Can you work these out from the model? Positions are in its coordinate system, mm. Face numbers are marked on the shaded views. A direction names the side the tool comes from. Round coordinates to 2 decimals unless told otherwise and drop trailing zeros. Order: outer loops, then holes, each group sorted by start corner. A loop starts at its lowest first (then second) coordinate and runs counter-clockwise, first axis right, second up. Notation, with made-up numbers: M 70.5,54 L 81.5,54 A23 ccw 81.5,84 Z; hole C 20.5,-8 d1. An arc over 180 degrees is marked long. Answer as a JSON object with one key per item and string values. Group by question number.
from build123d import *

# Parameters (mm, degrees)
CROQUIS1_W              = 44
CROQUIS1_H              = 25
SALIENTE_EXTRUIR2_DEPTH = 10
CROQUIS2_W              = 42
CROQUIS2_H              = 23
CORTAR_EXTRUIR1_DEPTH   = 9
CROQUIS3_W              = 1
CROQUIS3_H              = 2
SALIENTE_EXTRUIR3_DEPTH = 25
CROQUIS4_W              = 42
CROQUIS4_H              = 23
CORTAR_EXTRUIR2_DEPTH   = 28
CROQUIS5_W              = 1
CROQUIS5_H              = 23
CORTAR_EXTRUIR10_DEPTH  = 5
CROQUIS6_W              = 29.89343235
CROQUIS6_H              = 11.447342814
CORTAR_EXTRUIR11_DEPTH  = 1
CROQUIS7_W              = 31.003837105
CROQUIS7_H              = 9.868746677
CORTAR_EXTRUIR12_DEPTH  = 1
CROQUIS8_W              = 1
CROQUIS8_H              = 23
SALIENTE_EXTRUIR4_DEPTH = 5
CROQUIS9_W              = 8
CROQUIS9_H              = 4
CORTAR_EXTRUIR17_DEPTH  = 87
CROQUIS10_R             = 4
CORTAR_EXTRUIR19_DEPTH  = 10


with BuildPart() as part:
    # Croquis1 → Saliente-Extruir2 (new body)
    with BuildSketch(Plane(origin=(0, 0, 0), x_dir=(1, 0, 0), z_dir=(0, 1, 0))):
        Rectangle(CROQUIS1_W, CROQUIS1_H)
    extrude(amount=SALIENTE_EXTRUIR2_DEPTH)

    # Croquis2 → Cortar-Extruir1 (cut)
    with BuildSketch(Plane(origin=(0, 10, 0), x_dir=(1, 0, 0), z_dir=(0, 1, 0))):
        Rectangle(CROQUIS2_W, CROQUIS2_H)
    extrude(amount=-CORTAR_EXTRUIR1_DEPTH, mode=Mode.SUBTRACT)

    # Croquis3 → Saliente-Extruir3 (add)
    with BuildSketch(Plane.XY.offset(12.5)):
        Polygon((-23, 10), (-22, 10), (-16, 10), (-20, 13.5), (-20, 15), (-23, 15), align=None)
        Polygon((20, 13.5), (16, 10), (22, 10), (23, 10), (23, 15), (20, 15), align=None)
        with Locations((-22.5, 9)):
            Rectangle(CROQUIS3_W, CROQUIS3_H)
        with Locations((22.5, 9)):
            Rectangle(CROQUIS3_W, CROQUIS3_H)
    extrude(amount=-SALIENTE_EXTRUIR3_DEPTH)

    # Croquis4 → Cortar-Extruir2 (cut)
    with BuildSketch(Plane(origin=(0, 1, 0), x_dir=(1, 0, 0), z_dir=(0, 1, 0))):
        Rectangle(CROQUIS4_W, CROQUIS4_H)
    extrude(amount=CORTAR_EXTRUIR2_DEPTH, mode=Mode.SUBTRACT)

    # Croquis5 → Cortar-Extruir10 (cut)
    with BuildSketch(Plane(origin=(0, 15, 0), x_dir=(1, 0, 0), z_dir=(0, 1, 0))):
        with Locations((-21.5, 0)):
            Rectangle(CROQUIS5_W, CROQUIS5_H)
        with Locations((21.5, 0)):
            Rectangle(CROQUIS5_W, CROQUIS5_H)
    extrude(amount=-CORTAR_EXTRUIR10_DEPTH, mode=Mode.SUBTRACT)

    # Croquis6 → Cortar-Extruir11 (cut)
    with BuildSketch(Plane(origin=(23, 0, 0), x_dir=(0, 0, -1), z_dir=(1, 0, 0))):
        with Locations((-0.524699003, 11.114026003)):
            Rectangle(CROQUIS6_W, CROQUIS6_H)
    extrude(amount=-CORTAR_EXTRUIR11_DEPTH, mode=Mode.SUBTRACT)

    # Croquis7 → Cortar-Extruir12 (cut)
    with BuildSketch(Plane.ZY.offset(23)):
        with Locations((-0.729719636, 12.255463236)):
            Rectangle(CROQUIS7_W, CROQUIS7_H)
    extrude(amount=-CORTAR_EXTRUIR12_DEPTH, mode=Mode.SUBTRACT)

    # Croquis8 → Saliente-Extruir4 (add)
    with BuildSketch(Plane(origin=(0, 10, 0), x_dir=(1, 0, 0), z_dir=(0, 1, 0))):
        with Locations((-21.5, 0)):
            Rectangle(CROQUIS8_W, CROQUIS8_H)
        with Locations((21.5, 0)):
            Rectangle(CROQUIS8_W, CROQUIS8_H)
    extrude(amount=SALIENTE_EXTRUIR4_DEPTH)

    # Croquis9 → Cortar-Extruir17 (cut)
    with BuildSketch(Plane.ZY.offset(22)):
        with Locations((0, 5)):
            Rectangle(CROQUIS9_W, CROQUIS9_H)
    extrude(amount=-CORTAR_EXTRUIR17_DEPTH, mode=Mode.SUBTRACT)

    # Croquis10 → Cortar-Extruir19 (cut)
    with BuildSketch(Plane.XZ):
        with Locations(Location((0, 0, 0), (0, 0, 270))):
            Circle(CROQUIS10_R)
    extrude(amount=-CORTAR_EXTRUIR19_DEPTH, mode=Mode.SUBTRACT)


solid = part.part
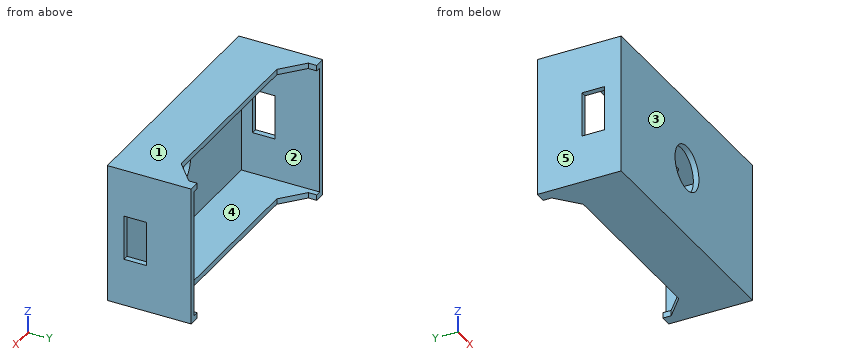
Item 1: If we mould it in two halves opening along X, with no side actions, what happens to the marked faces 3, 4 and 5? For each: +X half, -X half, draft (parallel to the pull), parting line (faces both ways), or undercut.
Item 2: On a 3-axis mill with a long thin cutter (end or side, diameter ignored), from which of +Z, -Z, +X, -X, +Y, -Y can I reach the whole of each face in a straight line? I mean the marked faces 1 and 2. Say none if no direction works.
Item 3: Suppose I cut it at A-A, the plane y = 7.75. Write out the boundary of the cut face in (x, z).
Item 4: Suppose I cut it at D-D, the plane y = 3.5. Write out the boundary of the cut face in (x, z).
Item 5: Suppose I cut it at B-B, the plane z = 0. Write out the boundary of the cut face in (x, y), and give its area (3 significant figures).
Item 6: I'm going to push flat-ended pins straight in: pin 1 Ø5 at (x, z) = (-15.5, 2.5) entering from +Y; pin 2 Ø0.8 at (x, z) = (3, -12) entering from +Y. Where does each tip first touch, or does it pass through?
Item 7: I need wall thicknesses on line 1 (X direction, y = 11.5, z = 6.75); line 2 (Z direction, x = 11, y = 8.5); line 3 (X direction, y = 0.3, z = 0). Which ranges of each line are inside material? Lowest first, please.
Item 8: Suppose I cut it at C-C, the plane x = 0. Write out the boundary of the cut face in (y, z), and give its area (3 significant figures).
Computed:
{
 "1": {"face 3": "draft", "face 4": "undercut", "face 5": "-X half"},
 "2": {"face 1": "+Z, +X, -X, +Y, -Y", "face 2": "+Y"},
 "3": {"outline": "M -22,-12.5 L 22,-12.5 L 22,12.5 L -22,12.5 Z; hole M -21,-11.5 L 21,-11.5 L 21,11.5 L -21,11.5 Z"},
 "4": {"outline": "M -22,-12.5 L 22,-12.5 L 22,-4 L 21,-4 L 21,-11.5 L -21,-11.5 L -21,-4 L -22,-4 Z; M -22,4 L -21,4 L -21,11.5 L 21,11.5 L 21,4 L 22,4 L 22,12.5 L -22,12.5 Z"},
 "5": {"outline": "M -22,0 L -4,0 L -4,1 L -21,1 L -21,3 L -22,3 Z; M -22,7 L -21,7 L -21,15 L -22,15 Z; M 4,0 L 22,0 L 22,3 L 21,3 L 21,1 L 4,1 Z; M 21,7 L 22,7 L 22,15 L 21,15 Z", "area": "56.0 mm^2"},
 "6": {"pin 1": "stops at y = 1", "pin 2": "stops at y = 10"},
 "7": {"line 1": "x = -22 to -21, 21 to 22", "line 2": "z = -12.5 to -11.5, 11.5 to 12.5", "line 3": "x = -22 to -4, 4 to 22"},
 "8": {"outline": "M 0,-12.5 L 10,-12.5 L 10,-11.5 L 1,-11.5 L 1,-4 L 0,-4 Z; M 0,4 L 1,4 L 1,11.5 L 10,11.5 L 10,12.5 L 0,12.5 Z", "area": "35.0 mm^2"}
}
